Read the model definition and answer for the solid it produces. Units are mm, in the model's axes. Face numbers are marked on the shaded views. A direction names the side the tool comes from. Coordinates: 2 decimals unless noted, no trailing zeros. Order: outer loops, then holes, each group sorted by start corner. A loop starts at its lowest first (then second) coordinate and runs counter-clockwise, first axis right, second up. Notation, with made-up numbers: (65, 55) -> (97, 55) arc R30 cw to (97, 85) -> close; hole circle Ø4 at (22.25, 82). An arc over 180 degrees is marked (long way). Answer as a JSON object with one key per item and string values. Group by question number.
1) Determine the mould class of the marked faces 4, 5 and 6 for opening direction X: released by +X, released by -X, zero draft, split by the parting line, or undercut.
2) Given pin 1 (4.5 mm diameter, centred on x = 76, z = 71, fed in from -Y); pin 2 (12 mm diameter, centred on y = 105.5, z = 39.5, fed in from +X); pin 3 (6 mm diameter, centred on y = 118, z = 66, fed in from -X), each flat-ended and moving along its own axis, determine where each tip first touches the part or whether it passes through.
3) Section B-B on y = -4.5 is taken. Determine the outline of the cut face in (x, z), and give its area (3 significant figures).
4) Section A-A on x = 47.5 is taken. Determine the outline of the cut face in (y, z).
5) A tool of negligible diameter and unlimited length cuts with its end or side. For the marked faces 1, 2 and 3, from which of +Z, -Z, +X, -X, +Y, -Y can it reach the whole face along a straight path? Write none if from no direction.
6) Section D-D on z = 14 is taken. Determine the outline of the cut face in (x, y), and give its area (3 significant figures).
7) Section C-C on x = 16 is taken. Determine the outline of the cut face in (y, z), and give its area (3 significant figures).
8) Consider L1, parallel to X at y = 61.5, z = 59; L2, parallel to Z at x = 35, y = 1.1; L3, parallel to Z at x = 27, y = 10. Determine where each line is inside the solid, lowest interval first.
from build123d import *

# Parameters (mm, degrees)
PAD_DEPTH         = 112
PAD001_DEPTH      = 112
SKETCH002_R       = 2.75
SKETCH002_W       = 48
SKETCH002_H       = 48
POCKET_DEPTH      = 32.001
PAD002_DEPTH      = 66
PAD002_DEPTH_BACK = 150
SKETCH004_W       = 28
SKETCH004_H       = 33
POCKET001_DEPTH   = 72.001
POCKET002_DEPTH   = 176.001
POCKET003_DEPTH   = 176.001
SKETCH007_R       = 5
PAD003_DEPTH      = 15
SKETCH008_R       = 5.25
PAD004_DEPTH      = 15
PAD005_DEPTH      = 176


with BuildPart() as part:
    # Sketch → Pad (new body)
    with BuildSketch(Plane.XY):
        with BuildLine():
            Line((-56, 32), (-56, 0))
            Line((56, 0), (-56, 0))
            Line((56, 32), (56, 0))
            ThreePointArc((56, 32), (53.171573, 30.828427), (52, 28))
            Line((52, 28), (52, 4))
            Line((52, 4), (-52, 4))
            Line((-52, 4), (-52, 28))
            ThreePointArc((-52, 28), (-53.171573, 30.828427), (-56, 32))
        make_face()
    extrude(amount=PAD_DEPTH)

    # Sketch001 (on Face8 of Pad) → Pad001 (join)
    with BuildSketch(Plane.YZ.offset(56)):
        with BuildLine():
            Line((0, 112), (32, 112))
            ThreePointArc((28, 108), (30.828427, 109.171573), (32, 112))
            Line((0, 108), (28, 108))
            Line((0, 108), (0, 112))
        make_face()
        with BuildLine():
            Line((0, 0), (32, 0))
            ThreePointArc((32, 0), (30.828427, 2.828427), (28, 4))
            Line((0, 4), (28, 4))
            Line((0, 0), (0, 4))
        make_face()
    extrude(amount=-PAD001_DEPTH)

    # Sketch002 (on Face13 of Pad001) → Pocket (cut, through all)
    with BuildSketch(Plane.XZ):
        with Locations((-35, 56)):
            Circle(SKETCH002_R)
        with Locations((35, 56)):
            Circle(SKETCH002_R)
        with Locations((0, 56)):
            Rectangle(SKETCH002_W, SKETCH002_H)
    extrude(amount=-POCKET_DEPTH, mode=Mode.SUBTRACT)

    # Sketch003 (on Face13 of Pocket) → Pad002 (join, two sides)
    with BuildSketch(Plane.XZ) as pad002_sk:
        with BuildLine():
            Line((56, 72), (56, 68))
            Line((56, 68), (84, 68))
            Line((84, 68), (84, 44))
            ThreePointArc((84, 44), (85.171573, 41.171573), (88, 40))
            Line((88, 72), (88, 40))
            Line((56, 72), (88, 72))
        make_face()
        with BuildLine():
            Line((-56, 72), (-56, 68))
            Line((-56, 68), (-84, 68))
            Line((-84, 68), (-84, 44))
            ThreePointArc((-88, 40), (-85.171573, 41.171573), (-84, 44))
            Line((-88, 72), (-88, 40))
            Line((-56, 72), (-88, 72))
        make_face()
    extrude(amount=PAD002_DEPTH)
    extrude(pad002_sk.sketch, amount=-PAD002_DEPTH_BACK)

    # Sketch004 (on Face18 of Pad002) → Pocket001 (cut, through all)
    with BuildSketch(Plane.XY.offset(72)):
        with Locations((70, -49.5)):
            Rectangle(SKETCH004_W, SKETCH004_H)
        with Locations((-70, -49.5)):
            Rectangle(SKETCH004_W, SKETCH004_H)
    extrude(amount=-POCKET001_DEPTH, mode=Mode.SUBTRACT)

    # Sketch005 (on Face39 of Pocket001) → Pocket002 (cut, through all)
    with BuildSketch(Plane.YZ.offset(88)):
        with BuildLine():
            Line((-66, 72), (-50, 72))
            ThreePointArc((-50, 72), (-61.313708, 67.313708), (-66, 56))
            Line((-66, 72), (-66, 56))
        make_face()
    extrude(amount=-POCKET002_DEPTH, mode=Mode.SUBTRACT)

    # Sketch006 (on Face39 of Pocket002) → Pocket003 (cut, through all)
    with BuildSketch(Plane.YZ.offset(88)):
        with BuildLine():
            Line((-50, 40), (-66, 40))
            Line((-66, 40), (-66, 56))
            ThreePointArc((-66, 56), (-61.313708, 44.686292), (-50, 40))
        make_face()
    extrude(amount=-POCKET003_DEPTH, mode=Mode.SUBTRACT)

    # Sketch007 (on Face39 of Pocket003) → Pad003 (join)
    with BuildSketch(Plane.YZ.offset(88)):
        with Locations((-50, 56)):
            Circle(SKETCH007_R)
    extrude(amount=PAD003_DEPTH)

    # Sketch008 (on Face53 of Pad003) → Pad004 (join)
    with BuildSketch(Plane(origin=(-88, 0, 0), x_dir=(0, -1, 0), z_dir=(-1, 0, 0))):
        with Locations((50, 56)):
            Circle(SKETCH008_R)
    extrude(amount=PAD004_DEPTH)

    # Sketch009 (on Face39 of Pad004) → Pad005 (join)
    with BuildSketch(Plane.YZ.offset(88)):
        with BuildLine():
            Line((150, 40), (150, 72))
            Line((150, 72), (118, 72))
            ThreePointArc((118, 72), (119.171573, 69.171573), (122, 68))
            Line((146, 68), (122, 68))
            Line((146, 68), (146, 44))
            ThreePointArc((146, 44), (147.171573, 41.171573), (150, 40))
        make_face()
    extrude(amount=-PAD005_DEPTH)


solid = part.part
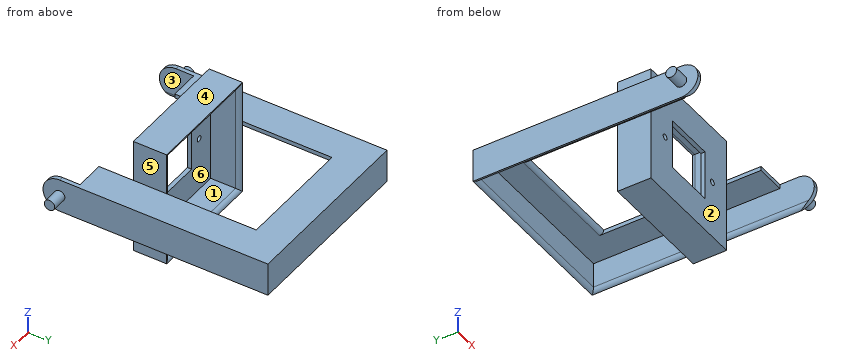
Worked answers:
{
 "1": {"face 4": "zero draft", "face 5": "released by +X", "face 6": "undercut"},
 "2": {"pin 1": "stops at y = -33", "pin 2": "stops at x = 88", "pin 3": "stops at x = -88"},
 "3": {"outline": "(-88, 40) arc R4 ccw to (-84, 44) -> (-84, 68) -> (-56, 68) -> (-56, 72) -> (-88, 72) -> close; (56, 68) -> (84, 68) -> (84, 44) arc R4 ccw to (88, 40) -> (88, 72) -> (56, 72) -> close", "area": "473 mm²"},
 "4": {"outline": "(0, 0) -> (32, 0) arc R4 ccw to (28, 4) -> (4, 4) -> (4, 108) -> (28, 108) arc R4 ccw to (32, 112) -> (0, 112) -> close; (118, 72) arc R4 ccw to (122, 68) -> (146, 68) -> (146, 44) arc R4 ccw to (150, 40) -> (150, 72) -> close"},
 "5": {"face 1": "+Y", "face 2": "+Z, -Z, -Y", "face 3": "-Z, -Y"},
 "6": {"outline": "(-56, 0) -> (56, 0) -> (56, 32) arc R4 ccw to (52, 28) -> (52, 4) -> (-52, 4) -> (-52, 28) arc R4 ccw to (-56, 32) -> close", "area": "665 mm²"},
 "7": {"outline": "(0, 0) -> (32, 0) arc R4 ccw to (28, 4) -> (4, 4) -> (4, 32) -> (0, 32) -> close; (0, 80) -> (4, 80) -> (4, 108) -> (28, 108) arc R4 ccw to (32, 112) -> (0, 112) -> close; (118, 72) arc R4 ccw to (122, 68) -> (146, 68) -> (146, 44) arc R4 ccw to (150, 40) -> (150, 72) -> close", "area": "706 mm²"},
 "8": {"L1": "x = -88 to -84, 84 to 88", "L2": "z = 0 to 53.25, 58.75 to 112", "L3": "z = 0 to 4, 108 to 112"}
}
